from build123d import *

# Parameters (mm, degrees)
SKETCH_1_W          = 9
SKETCH_1_H          = 9
EXTRUDE_1_DEPTH     = 582
SKETCH_2_W          = 7
SKETCH_2_H          = 7
CUT_EXTRUDE_1_DEPTH = 582
SKETCH_3_R          = 2.2
CUT_EXTRUDE_2_DEPTH = 582


with BuildPart() as part:
    # ｽｹｯﾁ1 → ﾎﾞｽ - 押し出し1 (new body)
    with BuildSketch(Plane.XY):
        Rectangle(SKETCH_1_W, SKETCH_1_H)
    extrude(amount=EXTRUDE_1_DEPTH)

    # ｽｹｯﾁ2 → ｶｯﾄ - 押し出し1 (cut)
    with BuildSketch(Plane.XY.offset(582)):
        Rectangle(SKETCH_2_W, SKETCH_2_H)
    extrude(amount=-CUT_EXTRUDE_1_DEPTH, mode=Mode.SUBTRACT)

    # ｽｹｯﾁ3 → ｶｯﾄ - 押し出し2 (cut)
    with BuildSketch(Plane(origin=(0, 4.5, 0), x_dir=(1, 0, 0), z_dir=(0, 1, 0))):
        with Locations((0, -5)):
            Circle(SKETCH_3_R)
        with Locations((0, -35)):
            Circle(SKETCH_3_R)
    extrude(amount=-CUT_EXTRUDE_2_DEPTH, mode=Mode.SUBTRACT)


solid = part.part
For this review, take the finished solid that the model builds, in its own axes (mm). Give positions to 0.01 mm unless a question says otherwise; leave off trailing zeros. Loops run counter-clockwise (first coordinate to the right, second up) from the corner with the lowest first, then second, coordinate; pieces in that order, holes last.
Item 1: Take a section at A-A, the plane z = 386. State the section outline as (x, y) points.
Item 2: Take a section at C-C, the plane y = 0. State the section outline as (x, z) points, and give its area (3 significant figures).
Item 3: For line 1 along Z through (x, y) = (0, 3.95); line 2 along X through (y, z) = (-3.8, 5); line 3 along Y through (x, z) = (0.75, 285), list the stretches that pass through material, from the lowest coordinate up.
Item 4: Take a section at B-B, the plane x = 0. State the section outline as (y, z) points.
Calculated:
1. outline: (-4.5, -4.5) - (4.5, -4.5) - (4.5, 4.5) - (-4.5, 4.5) - close; hole (-3.5, -3.5) - (3.5, -3.5) - (3.5, 3.5) - (-3.5, 3.5) - close
2. outline: (-4.5, 0) - (-3.5, 0) - (-3.5, 582) - (-4.5, 582) - close; (3.5, 0) - (4.5, 0) - (4.5, 582) - (3.5, 582) - close
2. area: 1,160 mm2
3. line 1: z = 0 to 2.8, 7.2 to 32.8, 37.2 to 582
3. line 2: x = -4.5 to -2.2, 2.2 to 4.5
3. line 3: y = -4.5 to -3.5, 3.5 to 4.5
4. outline: (-4.5, 0) - (-3.5, 0) - (-3.5, 2.8) - (-4.5, 2.8) - close; (-4.5, 7.2) - (-3.5, 7.2) - (-3.5, 32.8) - (-4.5, 32.8) - close; (-4.5, 37.2) - (-3.5, 37.2) - (-3.5, 582) - (-4.5, 582) - close; (3.5, 0) - (4.5, 0) - (4.5, 2.8) - (3.5, 2.8) - close; (3.5, 7.2) - (4.5, 7.2) - (4.5, 32.8) - (3.5, 32.8) - close; (3.5, 37.2) - (4.5, 37.2) - (4.5, 582) - (3.5, 582) - close
